Read the model definition and answer for the solid it produces. Units are mm, in the model's axes. A direction names the side the tool comes from. Coordinates: 2 decimals unless noted, no trailing zeros. Write each loop counter-clockwise with the first axis right and the second up, starting at its lowest first coordinate (ties: lowest second). Pieces come first, ordered by that corner, then holes.
(1) Section D-D on x = -4.5 is taken. Write down the section's boundary in (y, z), then the cut area to 3 significant figures.
(2) Section A-A on y = 0.75 is taken. Write down the section's boundary in (x, z).
(3) Which of the six approach directions +Z, -Z, +X, -X, +Y, -Y give full straight-line access (tool end or side, diameter ignored) to faces 4 (the flat face through (5.5, 10, 5)), 5 (the cylindrical face through (0.187, -8.498, 4.93))?
(4) Section B-B on z = 1.75 is taken. Write down the section's boundary in (x, y).
(5) Section C-C on x = 0 is taken. Write down the section's boundary in (y, z).
(6) The mould has two halves that part along X. Classify faces 1 (the flat face through (-5.5, 10, 5)), 2 (the flat face through (-6, 6, 0)), 3 (the flat face through (8.5, 10, 5)): +X half, -X half, draft (parallel to the pull), parting line (faces both ways), or undercut.
(7) Find the intervals of material crossed by probe 1 along X at (y, z) = (3.75, 3); probe 2 along X at (y, z) = (-1.5, 1); probe 3 along Y at (x, z) = (-0.25, 5), in increasing order.
Autodesk Inventor part; units mm, degrees
ref_plane "YZ Plane" through (0, 0, 0) normal (1, 0, 0) x (0, 1, 0)
ref_plane "XZ Plane" through (0, 0, 0) normal (0, 1, 0) x (-1, 0, 0)
ref_plane "XY Plane" through (0, 0, 0) normal (0, 0, 1) x (1, 0, 0)
sketch "Sketch1" plane through (0, 0, 0) normal (0, 0, 1) x (1, 0, 0)
  line L0 (-8.5, 0) -> (-5.5, 0)
  line L1 (-5.5, 0) -> (-5.5, 20)
  line L2 (-5.5, 20) -> (-8.5, 20)
  line L3 (-8.5, 20) -> (-8.5, 0)
  line L4 (8.5, 0) -> (5.5, 0)
  line L5 (5.5, 0) -> (5.5, 20)
  line L6 (5.5, 20) -> (8.5, 20)
  line L7 (8.5, 20) -> (8.5, 0)
  arc A0 (-5.5, 0) -> (5.5, 0) centre (0, 0) ccw
  arc A1 (-8.5, 0) -> (8.5, 0) centre (0, 0) ccw
  point P0 (0, 0)
  dimension "d0" = 3
  dimension "d1" = 3
  dimension "d2" = 5.5
  dimension "d3" = 5.5
  dimension "d4" = 20
  dimension "d5" = 20
extrude "Extrusion1" add sketch "Sketch1" along normal blind 10
properties part number "Plate_clip"
Response:
1. outline: (-7.21, 0) - (-3.16, 0) - (-3.16, 10) - (-7.21, 10) - close
1. area: 40.5 mm2
2. outline: (-8.5, 0) - (-5.5, 0) - (-5.5, 10) - (-8.5, 10) - close; (5.5, 0) - (8.5, 0) - (8.5, 10) - (5.5, 10) - close
3. face 4: +Z, -Z, +Y
3. face 5: +Z, -Z, -Y
4. outline: (-8.5, 0) arc R8.5 ccw to (8.5, 0) - (8.5, 20) - (5.5, 20) - (5.5, 0) arc R5.5 cw to (-5.5, 0) - (-5.5, 20) - (-8.5, 20) - close
5. outline: (-8.5, 0) - (-5.5, 0) - (-5.5, 10) - (-8.5, 10) - close
6. face 1: undercut
6. face 2: draft
6. face 3: +X half
7. probe 1: x = -8.5 to -5.5, 5.5 to 8.5
7. probe 2: x = -8.37 to -5.29, 5.29 to 8.37
7. probe 3: y = -8.5 to -5.49
